Can you work these out from the model? Positions are in its coordinate system, mm. A direction names the side the tool comes from. Round coordinates to 2 decimals unless told otherwise and drop trailing zeros. Use a Markdown table: item, result. Add a question column.
Q1. I need wall thicknesses on line 1 along Y through (x, z) = (45, 23); line 2 along Z through (x, y) = (87, -27.5); line 3 along Y through (x, z) = (38, 21). Which ranges of each line are inside material? Lowest first, please. Write a range as [from, to].
Q2. If we section it at A-A on x = 44: Give the number of separate pieces and of enclosed holes in the cut face, plus the area to 3 significant figures.
Q3. For faces 1 (the face through (19, -18, 21)), 2 (the face through (106.96, -10.45, -34.35)), 3 (the face through (69, 10, 6)), 4 (the face through (105.95, -9.07, 38.96)), 5 (the face through (70, 2, 0)), which set-ups out of +Z, -Z, +X, -X, +Y, -Y let a thin tool reach every point of the face, with its end or its side?
Q4. I'm going to push flat-ended pins straight in: pin 1 Ø12 at (y, z) = (-30.91, -8.28) entering from +X; pin 2 Ø5 at (y, z) = (-7, 27) entering from +X; pin 3 Ø6 at (y, z) = (23.5, -2) entering from +X; pin 4 Ø5 at (x, z) = (5.5, 14.5) entering from -Y. Where does each tip first touch, or does it pass through?
Q5. We'd pull the mould along Y, two halves only. Please class faces 6 (the face through (70, 25, 0)), 7 (the face through (69, 7, 15)), 8 (the face through (64.485, -11.943, -30.097)), 9 (the face through (69.8, -25.6, 27.4)): +Y half, -Y half, draft (parallel to the pull), parting line (faces both ways), or undercut.
```python
from build123d import *

# Parameters (mm, degrees)
REVOLVE1_ANGLE     = 270
CUT_EXTRUDE1_DEPTH = 151.069983674
SKETCH3_R          = 3.75
CUT_EXTRUDE2_DEPTH = 133.664991614
SKETCH5_R          = 30
CUT_EXTRUDE3_DEPTH = 151.069983674
CUT_EXTRUDE4_DEPTH = 151.06998382
CUT_EXTRUDE5_DEPTH = 10


with BuildPart() as part:
    # Sketch1 → Revolve1 (revolve)
    with BuildSketch(Plane.XY):
        with BuildLine():
            Line((47.5, 40), (50, 37.5))
            Line((50, 37.5), (89, 37.5))
            Line((89, 37.5), (91.5, 40))
            Line((91.5, 40), (120, 40))
            Line((120, 40), (120, 27))
            ThreePointArc((120, 27), (120.585786438, 25.585786438), (122, 25))
            Line((122, 25), (139, 25))
            Line((139, 25), (139, 0))
            Line((139, 0), (0, 0))
            Line((0, 0), (0, 25))
            Line((0, 25), (17, 25))
            ThreePointArc((17, 25), (18.414213562, 25.585786438), (19, 27))
            Line((19, 27), (19, 40))
            Line((19, 40), (47.5, 40))
        make_face()
    revolve(axis=Axis((0, 0, 0), (1, 0, 0)), revolution_arc=REVOLVE1_ANGLE)

    # Sketch2 → Cut-Extrude1 (cut, through all)
    with BuildSketch(Plane.ZY):
        with BuildLine():
            Line((0, 10), (12, 10))
            ThreePointArc((12, 10), (15, 7), (12, 4))
            Line((12, 4), (0, 4))
            ThreePointArc((0, 4), (-3, 7), (0, 10))
        make_face()
    extrude(amount=-CUT_EXTRUDE1_DEPTH, mode=Mode.SUBTRACT)

    # Sketch3 → Cut-Extrude2 (cut, through all)
    with BuildSketch(Plane(origin=(120, 0, 0), x_dir=(0, 0, -1), z_dir=(1, 0, 0))):
        with Locations((-8.282209443, 30.909626441)):
            Circle(SKETCH3_R)
        with Locations((30.909626441, -8.282209443)):
            Circle(SKETCH3_R)
        with Locations((22.627416998, -22.627416998)):
            Circle(SKETCH3_R)
        with Locations((8.282209443, -30.909626441)):
            Circle(SKETCH3_R)
        with Locations((-8.282209443, -30.909626441)):
            Circle(SKETCH3_R)
        with Locations((-22.627416998, -22.627416998)):
            Circle(SKETCH3_R)
        with Locations((-30.909626441, -8.282209443)):
            Circle(SKETCH3_R)
        with Locations((-30.909626441, 8.282209443)):
            Circle(SKETCH3_R)
        with Locations((-22.627416998, 22.627416998)):
            Circle(SKETCH3_R)
    extrude(amount=-CUT_EXTRUDE2_DEPTH, mode=Mode.SUBTRACT)

    # Sketch5 → Cut-Extrude3 (cut, through all)
    with BuildSketch(Plane(origin=(0, 0, 0), x_dir=(1, 0, 0), z_dir=(0, 1, 0))):
        with Locations((139, 40)):
            Circle(SKETCH5_R)
    extrude(amount=-CUT_EXTRUDE3_DEPTH, mode=Mode.SUBTRACT)

    # Sketch6 → Cut-Extrude4 (cut, through all)
    with BuildSketch(Plane(origin=(0, 0, 0), x_dir=(1, 0, 0), z_dir=(0, 1, 0))):
        with BuildLine():
            Line((104.531728645, 33.922313782), (109.45576741, 34.79055467))
            ThreePointArc((109.45576741, 34.79055467), (115.199399791, 21.73715713), (126.321452148, 12.810766389))
            Line((126.321452148, 12.810766389), (124.208360839, 8.279227454))
            ThreePointArc((124.208360839, 8.279227454), (111.23263309, 18.693349985), (104.531728645, 33.922313782))
        make_face()
    extrude(amount=-CUT_EXTRUDE4_DEPTH, mode=Mode.SUBTRACT)

    # Sketch8 → Cut-Extrude5 (cut)
    with BuildSketch(Plane.ZY):
        with BuildLine():
            Line((-19.364916731, -4), (-0.400463796, -4))
            Line((-0.400463796, -4), (3, -4))
            ThreePointArc((3, -4), (3.707106781, -3.707106781), (4, -3))
            Line((4, -3), (4, -0.903690713))
            ThreePointArc((4, -0.903690713), (4.292893219, -0.196583931), (5, 0.096309287))
            Line((5, 0.096309287), (19.979573146, 0.096309287))
            ThreePointArc((19.979573146, 0.096309287), (20.702478581, -0.21274373), (20.978551803, -0.948875248))
            ThreePointArc((20.978551803, -0.948875248), (2.174637981, -20.887100078), (-20.333162568, -5.25))
            ThreePointArc((-20.333162568, -5.25), (-20.155486146, -4.387627564), (-19.364916731, -4))
        make_face()
    extrude(amount=-CUT_EXTRUDE5_DEPTH, mode=Mode.SUBTRACT)


solid = part.part
```
Answer below:
| question | item | result |
|---|---|---|
| 1 | line 1 | [-32.73, -26.36], [-18.9, 18.9], [26.36, 32.73] |
| 1 | line 2 | [-25.5, -9.84], [-6.72, 6.72], [9.84, 25.5] |
| 1 | line 3 | [-34.04, -26.01], [-19.25, 19.25], [26.01, 34.04] |
| 2 | separate pieces | 1 |
| 2 | enclosed holes | 9 |
| 2 | area | 3,290 mm² |
| 3 | face 1 | -X |
| 3 | face 2 | +X, +Y, -Y |
| 3 | face 3 | -Z, +X, -X |
| 3 | face 4 | +X, -X |
| 3 | face 5 | -Z, +X, -X, +Y |
| 4 | pin 1 | x = 120.27 |
| 4 | pin 2 | x = 120.81 |
| 4 | pin 3 | x = 139 |
| 4 | pin 4 | y = -21.93 |
| 5 | face 6 | draft |
| 5 | face 7 | undercut |
| 5 | face 8 | undercut |
| 5 | face 9 | parting line |
